from build123d import *

# Parameters (mm, degrees)
SKETCH1_R           = 30.48
BOSS_EXTRUDE1_DEPTH = 9.525
SKETCH2_R           = 25.4
BOSS_EXTRUDE2_DEPTH = 12.7
SKETCH3_R           = 4.7625
CUT_EXTRUDE1_DEPTH  = 49.497540402


with BuildPart() as part:
    # Sketch1 → Boss-Extrude1 (new body)
    with BuildSketch(Plane.XY):
        with Locations(Location((0, 0, 0), (0, 0, 180))):
            Circle(SKETCH1_R)
    extrude(amount=BOSS_EXTRUDE1_DEPTH)

    # Sketch2 → Boss-Extrude2 (add)
    with BuildSketch(Plane.XY.offset(9.525)):
        Circle(SKETCH2_R)
    extrude(amount=BOSS_EXTRUDE2_DEPTH)

    # Sketch3 → Cut-Extrude1 (cut, through all)
    with BuildSketch(Plane.XY.offset(22.225)):
        Circle(SKETCH3_R)
    extrude(amount=-CUT_EXTRUDE1_DEPTH, mode=Mode.SUBTRACT)


solid = part.part
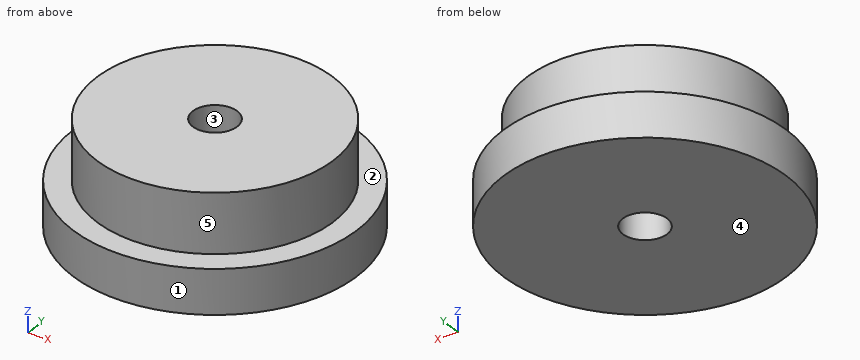
Can you work these out from the model? Positions are in its coordinate system, mm. Face numbers are marked on the shaded views. A direction names the side the tool comes from. Round coordinates to 2 decimals unless told otherwise and drop trailing zeros. Order: outer loops, then holes, each group sorted by start corner. A loop starts at its lowest first (then second) coordinate and runs counter-clockwise, first axis right, second up. Notation, with made-up numbers: (58.5, -24) -> (85.5, -24) arc R26 ccw to (85.5, -9) -> close; hole circle Ø2 at (88.25, 20.25). An arc over 180 degrees is marked (long way). Write each question's results on one line, items separated by ' | '. Start each with the question number.
Item 1: If we section it at A-A, the plane y = 0: Write out the boundary of the cut face in (x, z) (1 decimal).
Item 2: Please list where these lines run through material, in increasing order: L1, parallel to Y at x = 0, z = 10.75; L2, parallel to Y at x = 0, z = 4.5; L3, parallel to Z at x = 22.5, y = -20 (3 decimals).
Item 3: If we section it at D-D, the plane x = -16.5: Write out the boundary of the cut face in (y, z) (3 decimals), then the cut area to 3 significant figures.
Item 4: Thinking about a two-plate mould opening in Y: for the marked faces 1, 2 and 3, which applies, +Y half, -Y half, draft (parallel to the pull), parting line (faces both ways), or undercut?
Item 5: Which directions (+Z, -Z, +X, -X, +Y, -Y) give clear straight access to the entire face, cutting with the end or side of a thin tool? Please do the marked faces 4 and 5.
Item 6: Will these pins go through, and if not, where does the flat tip stop? pin 1 (3 mm diameter, centred on y = -7.5, z = 3, fed in from -X); pin 2 (6 mm diameter, centred on y = -16, z = 18.5, fed in from -X); pin 3 (6 mm diameter, centred on y = 12, z = 10, fed in from +X); pin 4 (12 mm diameter, centred on y = 0.5, z = 7.5, fed in from +X).
Item 7: If we section it at C-C, the plane z = 17: Write out the boundary of the cut face in (x, y) (1 decimal).
Results:
1) outline: (-30.5, 0) -> (-4.8, 0) -> (-4.8, 22.2) -> (-25.4, 22.2) -> (-25.4, 9.5) -> (-30.5, 9.5) -> close; (4.8, 0) -> (30.5, 0) -> (30.5, 9.5) -> (25.4, 9.5) -> (25.4, 22.2) -> (4.8, 22.2) -> close
2) L1: y = -25.4 to -4.76, 4.76 to 25.4 | L2: y = -30.48 to -4.76, 4.76 to 30.48 | L3: z = 0 to 9.525
3) outline: (-25.628, 0) -> (25.628, 0) -> (25.628, 9.525) -> (19.311, 9.525) -> (19.311, 22.225) -> (-19.311, 22.225) -> (-19.311, 9.525) -> (-25.628, 9.525) -> close | area: 979 mm2
4) face 1: parting line | face 2: draft | face 3: undercut
5) face 4: -Z, +X, -X, +Y, -Y | face 5: +Z
6) pin 1: stops at x = -29.88 | pin 2: stops at x = -21.82 | pin 3: stops at x = 29.11 | pin 4: stops at x = 30.48
7) outline: circle Ø50.8 at (0, 0); hole circle Ø9.5 at (0, 0)
